Can you work these out from the model? Positions are in its coordinate system, mm. A direction names the side the tool comes from. Round coordinates to 2 decimals unless told otherwise and drop trailing zeros. Order: outer loops, then holes, each group sorted by start corner. A loop starts at its lowest first (then second) coordinate and runs counter-clockwise, first axis right, second up.
Q1. If I drill on line 1 (X direction, y = 114, z = 7); line 2 (X direction, y = 23, z = 10.5); line 3 (Z direction, x = -33, y = 25), over which ranges is the centre line in solid material (lowest first)?
Q2. If we section it at A-A (y = 25): Please give me the cut outline in (x, z), plus the area to 3 significant figures.
Q3. If we section it at D-D (z = 34.5): Please give me the cut outline in (x, y).
Q4. If we section it at C-C (z = 13.5): Please give me the cut outline in (x, y), plus the area to 3 significant figures.
Q5. We'd pull the mould along X, two halves only. Please class faces 4 (the face through (-20, 130, 5)), 5 (the face through (-12.412, 95, 5)), 6 (the face through (-40, 41, 18)): pulls with the +X half, pulls with the -X half, needs draft (parallel to the pull), parting line crosses it, or undercut.
Q6. Will these pins go through, and if not, where does the flat tip stop? P1, Ø7.5, axis at y = 27, z = 50.5, coming from the -X side (3 decimals); P2, Ø13, axis at x = -8, z = 25, coming from the +Y side; P3, Ø18, axis at y = 25, z = 40, coming from the -X side; P4, Ø1.8, axis at x = -10.5, y = 34, coming from the +Z side.
Q7. If we section it at B-B (x = -20): Please give me the cut outline in (y, z), plus the area to 3 significant figures.
Q8. For faces 1 (the face through (-20.167, 67.414, 5.07)), 2 (the face through (-10, 24.7, 55.5)), 3 (the face through (-35, 50, 25)), which set-ups out of +Z, -Z, +X, -X, +Y, -Y let a thin tool reach every point of the face, with its end or its side?
Autodesk Fusion 360 part; units mm, degrees
sketch "Sketch1" plane through (0, 0, 0) normal (0, 1, 0) x (1, 0, 0)
  line L0 (0, 0) -> (-40, 0)
  line L1 (-40, 0) -> (-40, -40)
  line L2 (0, -40) -> (0, 0)
  line L3 (-40, -40) -> (-30, -40)
  line L4 (-30, -40) -> (-30, -10)
  line L5 (-30, -10) -> (-11.6065, -10)
  line L6 (-11.6065, -10) -> (-11.6065, -40)
  line L7 (-11.6065, -40) -> (0, -40)
  dimension "d6" = 40
  dimension "d7" = 40
  dimension "d8" = 10
  dimension "d9" = 11.6065
  dimension "d10" = 10
extrude "Extrude1" add sketch "Sketch1" along normal blind 130
sketch "Sketch2" plane through (-40, 0, 0) normal (-1, 0, 0) x (0, -1, 0)
  line L0 (0, 0) -> (0, 40)
  line L1 (0, 40) -> (-130, 40)
  line L2 (-130, 40) -> (-130, 0)
  line L3 (-130, 0) -> (0, 0)
  circle A0 centre (-25, 40) radius 15
  arc A1 (0, 40) -> (-50, 40) centre (-25, 40) ccw
  line L4 (-50, 40) -> (-50, 10)
  line L5 (-50, 10) -> (-130, 10)
  dimension "d13" = 50
  dimension "d14" = 30
  dimension "d15" = 25
  dimension "d16" = 30
extrude "Extrude2" add sketch "Sketch2" against normal blind 10 contours L1 A0 A1
extrude "Extrude3" cut sketch "Sketch2" against normal blind 10 contours L1 A0 | L1 A0
extrude "Extrude4" cut sketch "Sketch2" against normal blind 10 contours L1 L2 L4 L5
extrude "Extrude5" add sketch "Sketch2" against normal blind 10 contours L1 L2 L4 L5
sketch "Sketch3" plane through (-40, 0, 0) normal (-1, 0, 0) x (0, -1, 0)
  line L0 (-130, 10) -> (-130, 0)
  line L1 (-130, 0) -> (0, 0)
  line L2 (0, 0) -> (0, 40)
extrude "Extrude6" cut sketch "Sketch2" against normal blind 66.91 contours L1 L2 L4 L5
sketch "Sketch4" plane through (0, 0, 0) normal (1, 0, 0) x (0, 1, 0)
  line L0 (130, 10) -> (50, 10)
  line L1 (50, 10) -> (50, 40)
  line L2 (50, 40) -> (0, 40)
  line L3 (0, 40) -> (0, 0)
  line L4 (0, 0) -> (130, 0)
  line L5 (130, 0) -> (130, 10)
  circle A0 centre (25, 40) radius 15
  arc A1 (50, 40) -> (0, 40) centre (25, 40) ccw
  dimension "d27" = 50
  dimension "d28" = 30
extrude "Extrude7" cut sketch "Sketch4" against normal blind 10 contours L2 A0 A1 | L2 A0 | L2 A0
extrude "Extrude8" add sketch "Sketch4" against normal blind 10 contours L2 A0 A1
sketch "Sketch5" plane through (0, 0, 10) normal (0, 0, 1) x (-1, 0, 0)
  line L0 (30, -50) -> (30, 0)
  line L1 (30, 0) -> (11.6065, 0)
  line L2 (11.6065, 0) -> (11.6065, -50)
  line L3 (11.6065, -50) -> (0, -50)
  line L4 (0, -50) -> (0, -130)
  line L5 (0, -130) -> (40, -130)
  line L6 (40, -130) -> (40, -50)
  line L7 (40, -50) -> (30, -50)
  line L8 (12.4119, -75) -> (12.4119, -115)
  arc A0 (12.4119, -115) -> (27.5881, -115) centre (20, -115) ccw
  line L9 (27.5881, -115) -> (27.5881, -75)
  arc A1 (27.5881, -75) -> (12.4119, -75) centre (20, -75) ccw
  line L10 (20, -75) -> (20, -115) construction
  point P0 (20, -95)
  dimension "d33" = 40
extrude "Extrude9" cut sketch "Sketch5" against normal blind 34.041 contours L8 A0 L9 A1
Solution:
1. line 1: x = -40 to -27.59, -12.41 to 0
1. line 2: x = -40 to -30, -11.61 to 0
1. line 3: z = 0 to 25, 55 to 65
2. outline: (-40, 0) - (0, 0) - (0, 25) - (-10, 25) - (-10, 40) - (-11.61, 40) - (-11.61, 10) - (-30, 10) - (-30, 25) - (-40, 25) - close; (-40, 55) - (-30, 55) - (-30, 65) - (-40, 65) - close; (-10, 55) - (0, 55) - (0, 65) - (-10, 65) - close
2. area: 948 mm2
3. outline: (-40, 0) - (-30, 0) - (-30, 11.04) - (-40, 11.04) - close; (-40, 38.96) - (-30, 38.96) - (-30, 50) - (-40, 50) - close; (-11.61, 0) - (0, 0) - (0, 11.04) - (-10, 11.04) - (-10, 38.96) - (0, 38.96) - (0, 50) - (-11.61, 50) - close
4. outline: (-40, 0) - (-30, 0) - (-30, 50) - (-40, 50) - close; (-11.61, 0) - (0, 0) - (0, 50) - (-11.61, 50) - close
4. area: 1,080 mm2
5. face 4: needs draft
5. face 5: undercut
5. face 6: pulls with the -X half
6. P1: passes through
6. P2: stops at y = 50
6. P3: stops at x = -11.61
6. P4: stops at z = 63.6
7. outline: (0, 0) - (67.41, 0) - (67.41, 10) - (0, 10) - close; (122.59, 0) - (130, 0) - (130, 10) - (122.59, 10) - close
7. area: 748 mm2
8. face 1: +Z, -Z
8. face 2: +Z, +Y, -Y
8. face 3: +Z, +X, -X, +Y
